from build123d import *

# Parameters (mm, degrees)
F0_W     = 15
F0_H     = 15
F1_DEPTH = 30
F2_W     = 15
F2_H     = 15
F3_DEPTH = 2
F4_W     = 6.8767888099
F4_H     = 40
F5_DEPTH = 50
F6_W     = 32.9012749717
F6_H     = 6.8896561861
F7_DEPTH = 30
F8_R     = 1


with BuildPart() as f1:
    # F0 (on Top) → F1 (new body)
    with BuildSketch(Plane.XY):
        with Locations((42.5, 17.5)):
            Rectangle(F0_W, F0_H)
    extrude(amount=F1_DEPTH)



with BuildPart() as f1b:
    # F0 (on Top) → F1, piece 2 (new body)
    with BuildSketch(Plane.XY):
        with Locations((17.5, 17.5)):
            Rectangle(F0_W, F0_H)
    extrude(amount=F1_DEPTH)


with BuildPart() as f1c:
    # F0 (on Top) → F1, piece 3 (new body)
    with BuildSketch(Plane.XY):
        with Locations((17.5, 42.5)):
            Rectangle(F0_W, F0_H)
    extrude(amount=F1_DEPTH)


with BuildPart() as f1d:
    # F0 (on Top) → F1, piece 4 (new body)
    with BuildSketch(Plane.XY):
        with Locations((42.5, 42.5)):
            Rectangle(F0_W, F0_H)
    extrude(amount=F1_DEPTH)


with BuildPart() as f1_1:
    add(f1.part)

    add(f1b.part)  # F3 merges F1b

    add(f1c.part)  # F3 merges F1c

    add(f1d.part)  # F3 merges F1d
    # F2 (on face) → F3 (join)
    with BuildSketch(Plane.XY.offset(30)):
        with Locations((42.5, 17.5)):
            Rectangle(F2_W, F2_H)
        Polygon((10, 10), (35, 10), (35, 25), (50, 25), (50, 50), (10, 50), align=None)
    extrude(amount=F3_DEPTH)

    # F4 (on face) → F5 (join)
    with BuildSketch(Plane.XY.offset(32)):
        with Locations((13.4383944049, 30)):
            Rectangle(F4_W, F4_H)
    extrude(amount=F5_DEPTH)

    # F6 (on face) → F7 (cut)
    with BuildSketch(Plane(origin=(10, 0, 0), x_dir=(0, -1, 0), z_dir=(-1, 0, 0))):
        with Locations((-29.7453277744, 75.2560794353)):
            Rectangle(F6_W, F6_H)
    extrude(amount=-F7_DEPTH, mode=Mode.SUBTRACT)

    # F8
    f8_edges = [f1_1.edges().sort_by_distance(p)[0] for p in [
        (33.438394, 10, 32),
        (16.876789, 30, 32),
        (33.438394, 50, 32),
        (50, 30, 32),
        (16.876789, 10, 57),
        (16.876789, 30, 82),
        (16.876789, 50, 57),
        (16.876789, 29.745328, 78.700908),
        (16.876789, 46.195965, 75.256079),
        (16.876789, 29.745328, 71.811251),
        (16.876789, 13.29469, 75.256079),
    ]]
    fillet(f8_edges, radius=F8_R)


solid = f1_1.part
CAD build for the part. Positions are in the model's coordinates, mm. A direction names the side the tool comes from. Coordinates: 2 decimals unless noted, no trailing zeros. Order: outer loops, then holes, each group sorted by start corner. A loop starts at its lowest first (then second) coordinate and runs counter-clockwise, first axis right, second up.
Item 1: Band-saw the part on C-C on x = 46. List the corners of the cut face in (y, z).
Check sheet entries:
outline: (10, 0) - (25, 0) - (25, 30) - (35, 30) - (35, 0) - (50, 0) - (50, 31) arc R1 ccw to (49, 32) - (11, 32) arc R1 ccw to (10, 31) - close
Item 2: Band-saw the part on A-A on y = 33. List the corners of the cut face in (x, z), plus the area to 3 significant figures.
Check sheet entries:
outline: (10, 30) - (50, 30) - (50, 31) arc R1 ccw to (49, 32) - (17.88, 32) arc R1 cw to (16.88, 33) - (16.88, 70.81) arc R1 ccw to (15.88, 71.81) - (10, 71.81) - close; (10, 78.7) - (15.88, 78.7) arc R1 ccw to (16.88, 79.7) - (16.88, 81) arc R1 ccw to (15.88, 82) - (10, 82) - close
area: 376 mm2
Item 3: Band-saw the part on D-D on y = 39. List the corners of the cut face in (x, z).
Check sheet entries:
outline: (10, 0) - (25, 0) - (25, 30) - (35, 30) - (35, 0) - (50, 0) - (50, 31) arc R1 ccw to (49, 32) - (17.88, 32) arc R1 cw to (16.88, 33) - (16.88, 70.81) arc R1 ccw to (15.88, 71.81) - (10, 71.81) - close; (10, 78.7) - (15.88, 78.7) arc R1 ccw to (16.88, 79.7) - (16.88, 81) arc R1 ccw to (15.88, 82) - (10, 82) - close
Item 4: Band-saw the part on B-B on z = 10. List the corners of the cut face in (x, y).
Check sheet entries:
outline: (10, 10) - (25, 10) - (25, 25) - (10, 25) - close; (10, 35) - (25, 35) - (25, 50) - (10, 50) - close; (35, 10) - (50, 10) - (50, 25) - (35, 25) - close; (35, 35) - (50, 35) - (50, 50) - (35, 50) - close
Item 5: 3-axis set-ups, long thin cutter, end or side, ignore diameter. For faces 4 (the face through (42, 35, 15)), 5 (the face through (13, 13.295, 75)), 6 (the face through (33, 30, 32)), 7 (the face through (35, 42, 15)): which of +Z, -Z, +X, -X, +Y, -Y reach the whole face in a straight line?
Check sheet entries:
face 4: -Z, +X, -X
face 5: +X, -X
face 6: +Z, +X, +Y, -Y
face 7: -Z, +Y, -Y
Item 6: Pin check, flat tips, straight feed: pin 1 Ø8 at (x, y) = (26, 41) entering from -Z; pin 2 Ø5 at (x, z) = (21, 37.5) entering from +Y; pin 3 Ø3 at (y, z) = (20, 72) entering from +X; pin 4 Ø9.5 at (x, y) = (38, 27.5) entering from +Z. Stop position of each tip, or through.
Check sheet entries:
pin 1: stops at z = 0
pin 2: passes through
pin 3: stops at x = 16.88
pin 4: stops at z = 32
Item 7: Drill centre lines: L1, parallel to X at y = 24.5, z = 8.5; L2, parallel to Z at x = 16, y = 13.5. Where is each one in solid material? Low to high.
Check sheet entries:
L1: x = 10 to 25, 35 to 50
L2: z = 0 to 71.8, 78.71 to 81.99
Item 8: Two-plate mould, pull along X, no slides. Class faces 1 (the face through (17, 35, 15)), 2 (the face through (35, 17, 15)), 3 (the face through (16.877, 30, 51)): +X half, -X half, draft (parallel to the pull), parting line (faces both ways), or undercut.
Check sheet entries:
face 1: draft
face 2: undercut
face 3: +X half
